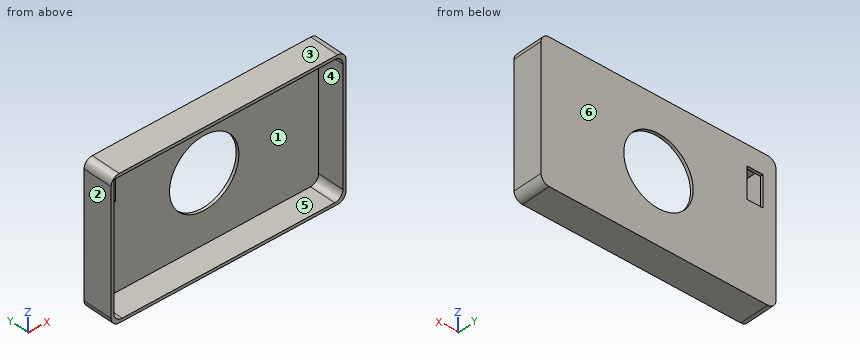
from build123d import *

# Parameters (mm, degrees)
F0_W     = 200.5350887775
F0_H     = 118.04754287
F1_DEPTH = 25.4
F2_T     = -2.54
F3_R     = 7
F4_W     = 13.4836062789
F4_H     = 26.3934414834
F5_DEPTH = 25
F6_R     = 29.6315052435
F7_DEPTH = 25


with BuildPart() as f1:
    # F0 (on Front) → F1 (new body)
    with BuildSketch(Plane.XZ):
        Rectangle(F0_W, F0_H)
    extrude(amount=F1_DEPTH)

    # F2
    f2_openings = [f1.faces().sort_by_distance(p)[0] for p in [
        (0, -25.4, 0),
    ]]
    offset(amount=F2_T, openings=f2_openings)

    # F3
    f3_edges = [f1.edges().sort_by_distance(p)[0] for p in [
        (-100.267544, -12.7, 59.023771),
        (100.267544, -12.7, 59.023771),
        (100.267544, -12.7, -59.023771),
        (-100.267544, -12.7, -59.023771),
        (97.727544, -13.97, 56.483771),
        (97.727544, -13.97, -56.483771),
        (-97.727544, -13.97, -56.483771),
    ]]
    fillet(f3_edges, radius=F3_R)

    # F4 (on face) → F5 (cut)
    with BuildSketch(Plane.XZ.offset(2.54)):
        with Locations((-82.4795104563, 28.8319671527)):
            Rectangle(F4_W, F4_H)
    extrude(amount=-F5_DEPTH, mode=Mode.SUBTRACT)

    # F6 (on face) → F7 (cut)
    with BuildSketch(Plane(origin=(0, 0, 0), x_dir=(-1, 0, 0), z_dir=(0, 1, 0))):
        Circle(F6_R)
    extrude(amount=-F7_DEPTH, mode=Mode.SUBTRACT)


solid = f1.part
Geometry check sheet. Reference: the model listing, model coordinates, mm. Face numbers are marked on the shaded views. A direction names the side the tool comes from. Give positions to 0.01 mm unless a question says otherwise; leave off trailing zeros. Order: outer loops, then holes, each group sorted by start corner. A loop starts at its lowest first (then second) coordinate and runs counter-clockwise, first axis right, second up.
1) Cross-section at D-D (z = 21). Record the boundary of the cut face in (x, y), then the cut area to 3 significant figures.
Results are:
outline: (-100.27, -25.4) - (-97.73, -25.4) - (-97.73, -2.54) - (-89.22, -2.54) - (-89.22, 0) - (-100.27, 0) - close; (-75.74, -2.54) - (-20.91, -2.54) - (-20.91, 0) - (-75.74, 0) - close; (20.91, -2.54) - (97.73, -2.54) - (97.73, -25.4) - (100.27, -25.4) - (100.27, 0) - (20.91, 0) - close
area: 485 mm2
2) Draft check along Z on the marked faces 1, 2, 3 and 4. Enter one of: released by +Z, released by -Z, zero draft, split by the parting line, or undercut.
Results are:
face 1: undercut
face 2: zero draft
face 3: released by +Z
face 4: undercut
3) Cross-section at C-C (y = -16). Record the boundary of the cut face in (x, z).
Results are:
outline: (-100.27, -52.02) arc R7 ccw to (-93.27, -59.02) - (93.27, -59.02) arc R7 ccw to (100.27, -52.02) - (100.27, 52.02) arc R7 ccw to (93.27, 59.02) - (-93.27, 59.02) arc R7 ccw to (-100.27, 52.02) - close; hole (-97.73, -49.48) arc R7 ccw to (-90.73, -56.48) - (90.73, -56.48) arc R7 ccw to (97.73, -49.48) - (97.73, 49.48) arc R7 ccw to (90.73, 56.48) - (-97.73, 56.48) - close
4) Tool access check on the marked faces 5 and 6. Record the directions out of +Z, -Z, +X, -X, +Y, -Y that give a thin tool (end or side, any length) a straight path to the whole face; none if there is none.
Results are:
face 5: -Y
face 6: +Z, -Z, +X, -X, +Y
5) Cross-section at A-A (z = 0). Record the boundary of the cut face in (x, y), then the cut area to 3 significant figures.
Results are:
outline: (-100.27, -25.4) - (-97.73, -25.4) - (-97.73, -2.54) - (-29.63, -2.54) - (-29.63, 0) - (-100.27, 0) - close; (29.63, -2.54) - (97.73, -2.54) - (97.73, -25.4) - (100.27, -25.4) - (100.27, 0) - (29.63, 0) - close
area: 475 mm2
6) Material ranges on probe 1 along Z at (x, y) = (0, -0.5); probe 2 along X at (y, z) = (-19.25, -6); probe 3 along Z at (x, y) = (-62, -17.5), recorded low to high.
Results are:
probe 1: z = -59.02 to -29.63, 29.63 to 59.02
probe 2: x = -100.27 to -97.73, 97.73 to 100.27
probe 3: z = -59.02 to -56.48, 56.48 to 59.02
7) Cross-section at B-B (x = 0). Record the boundary of the cut face in (y, z), then the cut area to 3 significant figures.
Results are:
outline: (-25.4, -59.02) - (0, -59.02) - (0, -29.63) - (-2.54, -29.63) - (-2.54, -56.48) - (-25.4, -56.48) - close; (-25.4, 56.48) - (-2.54, 56.48) - (-2.54, 29.63) - (0, 29.63) - (0, 59.02) - (-25.4, 59.02) - close
area: 265 mm2
